Autodesk Inventor part; units mm, degrees
ref_plane "YZ Plane" through (0, 0, 0) normal (1, 0, 0) x (0, 1, 0)
ref_plane "XZ Plane" through (0, 0, 0) normal (0, 1, 0) x (-1, 0, 0)
ref_plane "XY Plane" through (0, 0, 0) normal (0, 0, 1) x (1, 0, 0)
sketch "Sketch3" plane through (0, 0, 0) normal (0, 1, 0) x (-1, 0, 0)
  line L0 (-25.75, 13.25) -> (-25.75, -13.25)
  line L1 (-24.75, -14.25) -> (24.75, -14.25)
  line L2 (25.75, -13.25) -> (25.75, 13.25)
  line L3 (24.75, 14.25) -> (-24.75, 14.25)
  arc A0 (-25.75, -13.25) -> (-24.75, -14.25) centre (-24.75, -13.25) ccw
  arc A1 (-24.75, 14.25) -> (-25.75, 13.25) centre (-24.75, 13.25) ccw
  arc A2 (25.75, 13.25) -> (24.75, 14.25) centre (24.75, 13.25) ccw
  arc A3 (24.75, -14.25) -> (25.75, -13.25) centre (24.75, -13.25) ccw
  line L4 (24.75, -16.25) -> (-24.75, -16.25)
  arc A4 (-27.75, -13.25) -> (-24.75, -16.25) centre (-24.75, -13.25) ccw
  line L5 (-27.75, -13.25) -> (-27.75, 13.25)
  arc A5 (-24.75, 16.25) -> (-27.75, 13.25) centre (-24.75, 13.25) ccw
  line L6 (-24.75, 16.25) -> (24.75, 16.25)
  arc A6 (27.75, 13.25) -> (24.75, 16.25) centre (24.75, 13.25) ccw
  line L7 (27.75, 13.25) -> (27.75, -13.25)
  arc A7 (24.75, -16.25) -> (27.75, -13.25) centre (24.75, -13.25) ccw
  line L8 (21.75, -16.25) -> (21.75, -14.25)
  line L9 (27.75, -10.25) -> (25.75, -10.25)
  line L10 (25.75, 10.25) -> (27.75, 10.25)
  line L11 (21.75, 14.25) -> (21.75, 16.25)
  line L12 (-21.75, 14.25) -> (-21.75, 16.25)
  line L13 (-25.75, 10.25) -> (-27.75, 10.25)
  line L14 (-25.75, -10.25) -> (-27.75, -10.25)
  line L15 (-21.75, -16.25) -> (-21.75, -14.25)
  line L16 (-21.75, -14.25) -> (-17.75, -14.25)
  arc A8 (-17.75, -14.25) -> (-21.75, -16.25) centre (-15.3911, -23.9678) ccw
  line L17 (-21.75, 14.25) -> (-17.75, 14.25)
  arc A9 (-21.75, 16.25) -> (-17.75, 14.25) centre (-15.3911, 23.9678) ccw
  line L18 (-25.75, -10.25) -> (-25.75, -6.2495)
  line L19 (-25.75, 10.25) -> (-25.75, 6.25)
  arc A10 (-27.75, -10.25) -> (-25.75, -6.2495) centre (-35.468, -3.8913) ccw
  arc A11 (-25.75, 6.25) -> (-27.75, 10.25) centre (-35.4678, 3.8911) ccw
  line L20 (25.75, -10.25) -> (25.75, -6.2495)
  arc A12 (25.75, -6.2495) -> (27.75, -10.25) centre (35.468, -3.8913) ccw
  line L21 (25.75, 10.25) -> (25.75, 6.25)
  arc A13 (27.75, 10.25) -> (25.75, 6.25) centre (35.4678, 3.8911) ccw
  point P0 (0, 0)
  point P1 (0, 0)
  point P2 (-25.75, 14.25)
  point P3 (-25.75, -14.25)
  point P4 (25.75, -14.25)
  point P5 (21.75, 15.25)
  point P6 (-26.75, 10.25)
  dimension "d8" = 28.5
  dimension "d9" = 51.5
  dimension "d10" = 14.25
  dimension "d11" = 25.75
  dimension "d12" = 1
  dimension "d13" = 2
  dimension "d14" = 3
  dimension "d15" = 3
  dimension "d16" = 3
  dimension "d17" = 3
  dimension "d18" = 3
  dimension "d19" = 3
  dimension "d20" = 3
  dimension "d21" = 3
  dimension "d22" = 4
  dimension "d23" = 10
  dimension "d24" = 10
  dimension "d25" = 4
  dimension "d26" = 10
  dimension "d27" = 10
  dimension "d28" = 10
  dimension "d29" = 10
extrude "Extrusion2" add sketch "Sketch3" along normal blind 3 contours L0 L13 L5 A5 L6 L12 L3 A1 | L0 A11 L13 | L12 A9 L3 | L0 L14 A10 | L14 L0 A0 L1 L15 L4 A4 L5 | L11 L6 A6 L7 L10 L2 A2 L3 | L15 L1 A8 | L8 L1 A3 L2 L9 L7 A7 L4 | L10 A13 L2 | L9 L2 A12
sketch "Sketch4" plane through (0, 0, 0) normal (0, -1, 0) x (1, 0, 0)
  line L0 (-27.75, -13.25) -> (-27.75, -10.25)
  arc A0 (-27.75, -13.25) -> (-24.75, -16.25) centre (-24.75, -13.25) ccw
  line L1 (-21.75, -16.25) -> (-24.75, -16.25)
  line L2 (-24.75, 16.25) -> (-21.75, 16.25)
  arc A1 (-24.75, 16.25) -> (-27.75, 13.25) centre (-24.75, 13.25) ccw
  line L3 (-27.75, 10.25) -> (-27.75, 13.25)
  line L4 (21.75, 16.25) -> (24.75, 16.25)
  arc A2 (27.75, 13.25) -> (24.75, 16.25) centre (24.75, 13.25) ccw
  line L5 (27.75, 13.25) -> (27.75, 10.25)
  line L6 (27.75, -10.25) -> (27.75, -13.25)
  arc A3 (24.75, -16.25) -> (27.75, -13.25) centre (24.75, -13.25) ccw
  line L7 (24.75, -16.25) -> (21.75, -16.25)
  line L8 (-21.75, -16.25) -> (21.75, -16.25)
  line L9 (-27.75, -10.25) -> (-27.75, 10.25)
  line L10 (-25.75, -6.2495) -> (-25.75, -13.25)
  line L11 (-21.75, 16.25) -> (-21.75, 14.25)
  arc A4 (17.75, 14.25) -> (21.75, 16.25) centre (15.3911, 23.9678) ccw
  line L12 (-21.75, 16.25) -> (21.75, 16.25)
  arc A5 (25.75, -6.2495) -> (27.75, -10.25) centre (35.468, -3.8913) ccw
  line L13 (27.75, 10.25) -> (27.75, -10.25)
  point P0 (0, 0)
extrude "Extrusion3" add sketch "Sketch4" along normal blind 1.5
sketch "Sketch5" plane through (0, 0, 0) normal (0, 1, 0) x (1, 0, 0)
  line L0 (-21.75, -14.25) -> (-24.75, -14.25)
  line L1 (-24.75, -14.25) -> (-24.75, -12.05)
  line L2 (-24.75, -12.05) -> (-23.55, -12.05)
  line L3 (-24.75, 14.25) -> (-21.75, 14.25)
  line L4 (-24.75, 14.25) -> (-24.75, 12.05)
  line L5 (-24.75, 12.05) -> (-23.55, 12.05)
  arc A0 (25.75, 13.25) -> (24.75, 14.25) centre (24.75, 13.25) ccw
  line L6 (24.75, 14.25) -> (24.75, 12.05)
  line L7 (24.75, 12.05) -> (23.55, 12.05)
  arc A1 (24.75, -14.25) -> (25.75, -13.25) centre (24.75, -13.25) ccw
  line L8 (24.75, -14.25) -> (24.75, -12.05)
  line L9 (24.75, -12.05) -> (23.55, -12.05)
  point P0 (0, 0)
  dimension "d34" = 2.2
  dimension "d35" = 1.2
  dimension "d36" = 2.2
  dimension "d37" = 2.2
  dimension "d38" = 1.2
  dimension "d39" = 2.2
hole "Hole1" at (-23.55, 0, 12.05) at (-23.55, 0, -12.05) at (23.55, 0, -12.05) at (23.55, 0, 12.05) direction (0, -1, 0) diameter 3 end through all
sketch "Sketch6" plane through (0, 3, 0) normal (0, 1, 0) x (1, 0, 0)
  line L0 (25.75, -6.25) -> (25.75, 6.152)
  line L1 (24.75, -14.25) -> (17.75, -14.25)
  line L2 (17.75, -14.25) -> (-21.75, -14.25)
  arc A0 (-25.75, 6.2495) -> (-27.75, 10.25) centre (-35.468, 3.8913) ccw
  line L3 (-25.75, -6.25) -> (-25.75, 6.2495)
  line L4 (-24.75, 14.25) -> (-21.75, 14.25)
  line L5 (-21.75, 14.25) -> (17.75, 14.25)
  line L6 (25.75, -6.25) -> (25.75, -13.25)
  arc A1 (24.75, -16.25) -> (27.75, -13.25) centre (24.75, -13.25) ccw
  arc A2 (25.75, -10.25) -> (27.75, -13.25) centre (29, -10.25) ccw
  line L7 (25.75, -6.25) -> (25.75, -13.25)
  line L8 (25.75, 13.25) -> (25.75, 6.2495)
  arc A3 (27.75, 10.25) -> (25.75, 6.2495) centre (35.468, 3.8913) ccw
  line L9 (27.75, 10.25) -> (27.75, 13.25)
  line L10 (17.75, 14.25) -> (24.75, 14.25)
  arc A4 (17.75, 14.25) -> (21.75, 16.25) centre (15.3911, 23.9678) ccw
  line L11 (24.75, 16.25) -> (21.75, 16.25)
  line L12 (-27.75, 13.25) -> (-27.75, 10.25)
  arc A5 (-25.75, 6.2495) -> (-27.75, 10.25) centre (-35.468, 3.8913) ccw
  line L13 (-25.75, 6.2495) -> (-25.75, 13.25)
  line L14 (-21.75, 14.25) -> (-21.75, 16.25)
  line L15 (-21.75, 16.25) -> (-24.75, 16.25)
  arc A6 (-27.75, -10.25) -> (-25.75, -6.25) centre (-35.4678, -3.8911) ccw
  line L16 (-25.75, -13.25) -> (-25.75, -6.25)
  line L17 (-27.75, -10.25) -> (-27.75, -13.25)
  arc A7 (-27.75, -13.25) -> (-24.75, -16.25) centre (-24.75, -13.25) ccw
  line L18 (-24.75, -16.25) -> (-21.75, -16.25)
  line L19 (-21.75, -16.25) -> (-21.75, -14.25)
  arc A8 (21.75, -16.25) -> (17.75, -14.25) centre (15.3911, -23.9678) ccw
  line L20 (21.75, -16.25) -> (21.75, -14.25)
  arc A9 (-27.75, -13.25) -> (-25.75, -10.4161) centre (-28.7577, -10.4161) ccw
  arc A10 (27.75, 13.25) -> (25.75, 9.6748) centre (29.9455, 9.6748) ccw
  arc A11 (-25.75, 10.3378) -> (-27.75, 13.25) centre (-28.8703, 10.3378) ccw
  line L21 (21.75, 16.25) -> (21.75, 14.25)
  line L22 (27.75, -13.25) -> (27.75, -10.25)
  arc A12 (25.75, -6.25) -> (27.75, -10.25) centre (35.4678, -3.8911) ccw
  point P0 (0, 0)
extrude "Extrusion4" cut sketch "Sketch6" against normal blind 3
sketch "Sketch7" plane through (0, 3, 0) normal (0, 1, 0) x (1, 0, 0)
  arc A0 (25.75, -10.25) -> (27.75, -13.25) centre (29, -10.25) ccw
  arc A1 (24.75, -16.25) -> (27.75, -13.25) centre (24.75, -13.25) ccw
  arc A2 (24.75, -14.25) -> (25.75, -13.25) centre (24.75, -13.25) ccw
  line L0 (25.75, -10.25) -> (25.75, -13.25)
  line L1 (24.75, -14.25) -> (21.75, -14.25)
  line L2 (21.75, -14.25) -> (21.75, -16.25)
  line L3 (21.75, -16.25) -> (24.75, -16.25)
  line L4 (-21.75, -14.25) -> (-24.75, -14.25)
  line L5 (-21.75, -16.25) -> (-21.75, -14.25)
  line L6 (-24.75, -16.25) -> (-21.75, -16.25)
  arc A3 (-27.75, -13.25) -> (-24.75, -16.25) centre (-24.75, -13.25) ccw
  arc A4 (-27.75, -13.25) -> (-25.75, -10.4161) centre (-28.7577, -10.4161) ccw
  line L7 (-25.75, -13.25) -> (-25.75, -10.4161)
  arc A5 (-25.75, -13.25) -> (-24.75, -14.25) centre (-24.75, -13.25) ccw
  arc A6 (-25.75, 10.3378) -> (-27.75, 13.25) centre (-28.8703, 10.3378) ccw
  line L8 (-25.75, 10.3378) -> (-25.75, 13.25)
  arc A7 (-24.75, 14.25) -> (-25.75, 13.25) centre (-24.75, 13.25) ccw
  line L9 (-24.75, 14.25) -> (-21.75, 14.25)
  line L10 (-21.75, 14.25) -> (-21.75, 16.25)
  line L11 (-21.75, 16.25) -> (-24.75, 16.25)
  arc A8 (-24.75, 16.25) -> (-27.75, 13.25) centre (-24.75, 13.25) ccw
  arc A9 (27.75, 13.25) -> (24.75, 16.25) centre (24.75, 13.25) ccw
  line L12 (24.75, 16.25) -> (21.75, 16.25)
  line L13 (21.75, 16.25) -> (21.75, 14.25)
  line L14 (21.75, 14.25) -> (24.75, 14.25)
  arc A10 (25.75, 13.25) -> (24.75, 14.25) centre (24.75, 13.25) ccw
  line L15 (25.75, 13.25) -> (25.75, 9.6748)
  arc A11 (27.75, 13.25) -> (25.75, 9.6748) centre (29.9455, 9.6748) ccw
  point P0 (0, 0)
extrude "Extrusion5" add sketch "Sketch7" along normal blind 6.25
Verification items for the finished model (mm, model axes). A direction names the side the tool comes from. Give positions to 0.01 mm unless a question says otherwise; leave off trailing zeros. Loops run counter-clockwise (first coordinate to the right, second up) from the corner with the lowest first, then second, coordinate; pieces in that order, holes last.
1. Cross-section at B-B on y = 6.75. Record the cut outline in (x, z), and give its area (3 significant figures).
Derived:
outline: (-27.75, -13.25) arc R3 ccw to (-24.75, -16.25) - (-21.75, -16.25) - (-21.75, -14.25) - (-24.75, -14.25) arc R1 cw to (-25.75, -13.25) - (-25.75, -10.34) arc R3.12 cw to start; (-27.75, 13.25) arc R3.01 cw to (-25.75, 10.42) - (-25.75, 13.25) arc R1 cw to (-24.75, 14.25) - (-21.75, 14.25) - (-21.75, 16.25) - (-24.75, 16.25) arc R3 ccw to start; (21.75, -16.25) - (24.75, -16.25) arc R3 ccw to (27.75, -13.25) arc R4.2 cw to (25.75, -9.67) - (25.75, -13.25) arc R1 cw to (24.75, -14.25) - (21.75, -14.25) - close; (21.75, 14.25) - (24.75, 14.25) arc R1 cw to (25.75, 13.25) - (25.75, 10.25) arc R3.25 cw to (27.75, 13.25) arc R3 ccw to (24.75, 16.25) - (21.75, 16.25) - close
area: 56.0 mm2
2. Cross-section at D-D on z = -12.05. Record the cut outline in (x, y).
Derived:
outline: (-27.75, -1.5) - (-25.05, -1.5) - (-25.05, 0) - (-25.75, 0) - (-25.75, 9.25) - (-26.26, 9.25) - (-26.26, 0) - (-27.75, 0) - close; (-22.05, -1.5) - (22.05, -1.5) - (22.05, 0) - (-22.05, 0) - close; (25.05, -1.5) - (27.75, -1.5) - (27.75, 0) - (26.49, 0) - (26.49, 9.25) - (25.75, 9.25) - (25.75, 0) - (25.05, 0) - close
3. Cross-section at C-C on z = 12.05. Record the cut outline in (x, y).
Derived:
outline: (-27.75, -1.5) - (-25.05, -1.5) - (-25.05, 0) - (-25.75, 0) - (-25.75, 9.25) - (-26.23, 9.25) - (-26.23, 0) - (-27.75, 0) - close; (-22.05, -1.5) - (22.05, -1.5) - (22.05, 0) - (-22.05, 0) - close; (25.05, -1.5) - (27.75, -1.5) - (27.75, 0) - (26.29, 0) - (26.29, 9.25) - (25.75, 9.25) - (25.75, 0) - (25.05, 0) - close
4. Tool access check on faces 5 (the cylindrical face through (-26.85, 3.95, -15.39)), 6 (the flat face through (23, 5, 14.25)), 7 (the cylindrical face through (-26.28, 4.69, -12.08)), 8 (the flat face through (21.75, 5, -15)). Record the directions out of +Z, -Z, +X, -X, +Y, -Y that give a thin tool (end or side, any length) a straight path to the whole face; none if there is none.
Derived:
face 5: -Z, -X, +Y, -Y
face 6: +Y
face 7: -X, +Y
face 8: +Z, -Z, +Y
5. Release check for a two-part mould opening along X. For faces 1 (the cylindrical face through (-22.086, -0.76, -12.375)), 2 (the cylindrical face through (-26.315, 4.69, 12.171)), 3 (the flat face through (-25, 9.25, -15)), 4 (the cylindrical face through (26.85, 3.95, 15.39)) record: +X half, -X half, draft (parallel to the pull), parting line (faces both ways), or undercut.
Derived:
face 1: undercut
face 2: -X half
face 3: draft
face 4: +X half
6. Go/stop test with flat-tipped pins: P1, Ø6, axis at x = -13.5, y = 1, coming from the -Z side; P2, Ø2, axis at y = 8, z = 12, coming from the +X side; P3, Ø2.5, axis at y = 5.5, z = -11.5, coming from the +X side; P4, Ø0.9, axis at y = 3.5, z = 11.5, coming from the +X side. Record where each tip stops, or that it passes through.
Derived:
P1: stops at z = -16.25
P2: stops at x = 27.27
P3: stops at x = 27.09
P4: stops at x = 26.23
7. Material ranges on probe 1 along Z at (x, y) = (-23.55, -0.95); probe 2 along X at (y, z) = (-1, 12.05); probe 3 along Z at (x, y) = (24, 2.75), recorded low to high.
Derived:
probe 1: z = -16.25 to -13.55, -10.55 to 10.55, 13.55 to 16.25
probe 2: x = -27.75 to -25.05, -22.05 to 22.05, 25.05 to 27.75
probe 3: z = -16.25 to -14.25, 14.25 to 16.25
8. Cross-section at A-A on x = -23.55. Record the cut outline in (y, z).
Derived:
outline: (-1.5, -16.25) - (9.25, -16.25) - (9.25, -14.25) - (0, -14.25) - (0, -13.55) - (-1.5, -13.55) - close; (-1.5, -10.55) - (0, -10.55) - (0, 10.55) - (-1.5, 10.55) - close; (-1.5, 13.55) - (0, 13.55) - (0, 14.25) - (9.25, 14.25) - (9.25, 16.25) - (-1.5, 16.25) - close
